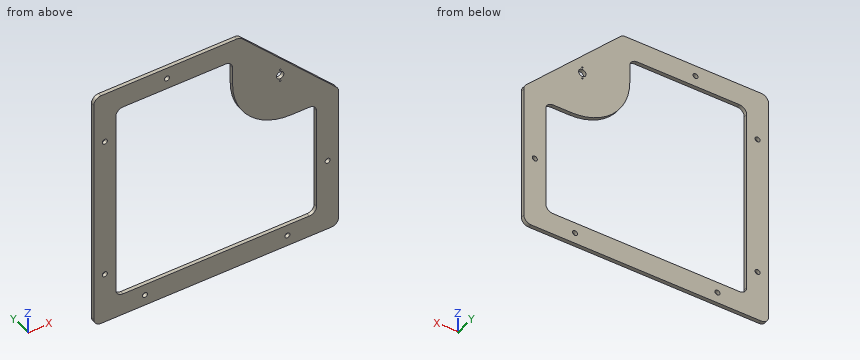
```python
from build123d import *

# Parameters (mm, degrees)
SKETCH1_W                = 425.45
SKETCH1_H                = 425.45
BOSS_EXTRUDE1_DEPTH      = 3.175
CUT_EXTRUDE1_DEPTH       = 301.90558943
SKETCH3_R                = 6.477
SKETCH3_R_2              = 1.27
CUT_EXTRUDE2_DEPTH       = 301.90558943
F_0_332_DIAMETER_HOLE1_D = 8.8392
CUT_EXTRUDE3_DEPTH       = 301.90558943
FILLET1_R                = 12.7
FILLET2_R                = 101.6


with BuildPart() as part:
    # Sketch1 → Boss-Extrude1 (new, symmetric)
    with BuildSketch(Plane(origin=(0, 0, 0), x_dir=(1, 0, 0), z_dir=(0, 1, 0))):
        Rectangle(SKETCH1_W, SKETCH1_H)
    extrude(amount=BOSS_EXTRUDE1_DEPTH, both=True)

    # Sketch2 → Cut-Extrude1 (cut, through all)
    with BuildSketch(Plane(origin=(0, 3.175, 0), x_dir=(1, 0, 0), z_dir=(0, 1, 0))):
        Polygon((212.725, -212.725), (212.725, -41.275), (41.275, -212.725), align=None)
    extrude(amount=-CUT_EXTRUDE1_DEPTH, mode=Mode.SUBTRACT)

    # Sketch3 → Cut-Extrude2 (cut, through all)
    with BuildSketch(Plane(origin=(0, 3.175, 0), x_dir=(1, 0, 0), z_dir=(0, 1, 0))):
        with Locations(Location((111.125, -111.125, 0), (0, 0, 270))):
            Circle(SKETCH3_R)
        with Locations(Location((111.125, -100.7999, 0), (0, 0, 270))):
            Circle(SKETCH3_R_2)
        with Locations(Location((111.125, -121.4501, 0), (0, 0, 270))):
            Circle(SKETCH3_R_2)
    extrude(amount=-CUT_EXTRUDE2_DEPTH, mode=Mode.SUBTRACT)

    # 0.332_ Diameter Hole1 (through all)
    with Locations(Plane(origin=(0, 3.175, 0), x_dir=(1, 0, 0), z_dir=(0, 1, 0))):
        with Locations((-85.725, -193.675), (-193.675, -123.825), (-193.675, 123.825), (-123.825, 193.675), (123.825, 193.675), (193.675, 85.725)):
            Hole(F_0_332_DIAMETER_HOLE1_D / 2)

    # Sketch6 → Cut-Extrude3 (cut, through all)
    with BuildSketch(Plane(origin=(0, 3.175, 0), x_dir=(1, 0, 0), z_dir=(0, 1, 0))):
        Polygon((174.625, 174.625), (174.625, -28.575), (28.575, -28.575), (28.575, -174.625), (-174.625, -174.625), (-174.625, 174.625), align=None)
    extrude(amount=-CUT_EXTRUDE3_DEPTH, mode=Mode.SUBTRACT)

    # Fillet1
    fillet1_edges = [part.edges().sort_by_distance(p)[0] for p in [
        (41.275, 0, 212.725),
        (212.725, 0, 41.275),
        (-212.725, 0, 212.725),
        (-212.725, 0, -212.725),
        (-174.625, 0, -174.625),
        (212.725, 0, -212.725),
        (174.625, 0, -174.625),
        (174.625, 0, 28.575),
        (28.575, 0, 174.625),
        (-174.625, 0, 174.625),
    ]]
    fillet(fillet1_edges, radius=FILLET1_R)

    # Fillet2
    fillet2_edges = [part.edges().sort_by_distance(p)[0] for p in [
        (28.575, 0, 28.575),
    ]]
    fillet(fillet2_edges, radius=FILLET2_R)


solid = part.part
```
Model file for the job. Use its own axes, mm. Give positions to 0.01 mm unless a question says otherwise; leave off trailing zeros. Order: outer loops, then holes, each group sorted by start corner. A loop starts at its lowest first (then second) coordinate and runs counter-clockwise, first axis right, second up.
1) Saw through at B-B, the plane z = 8. Write the cut outline in (x, y) (3 decimals).
2) Pin check, flat tips, straight feed: pin 1 (3 mm diameter, centred on y = -1.5, z = 41.5, fed in from +X); pin 2 (2 mm diameter, centred on x = 41, y = 0, fed in from +Z); pin 3 (1.5 mm diameter, centred on x = 111.12, z = 100.8, fed in from +Y); pin 4 (1 mm diameter, centred on y = -1, z = 100.5, fed in from +X). Stop position of each tip, or through.
3) Saw through at C-C, the plane y = 0.75. Count the separate pieces of the cut face and the enclosed holes in it, then the cut area to 3 significant figures.
4) Saw through at A-A, the plane x = -35.5. Write the cut outline in (y, z) (3 decimals).
5) Wall check: probe 1 along Z at (x, y) = (-85, 1) (3 decimals); probe 2 along X at (y, z) = (-2, -16) (3 decimals). Give the ranges that are in metal, low to high.
Computed:
1. outline: (-212.725, -3.175) - (-174.625, -3.175) - (-174.625, 3.175) - (-212.725, 3.175) - close; (174.625, -3.175) - (212.725, -3.175) - (212.725, 3.175) - (174.625, 3.175) - close
2. pin 1: stops at x = 212.08
2. pin 2: stops at z = 212.08
2. pin 3: passes through
2. pin 4: stops at x = 154
3. separate pieces: 1
3. enclosed holes: 10
3. area: 63,000 mm2
4. outline: (-3.175, -212.725) - (3.175, -212.725) - (3.175, -174.625) - (-3.175, -174.625) - close; (-3.175, 174.625) - (3.175, 174.625) - (3.175, 212.725) - (-3.175, 212.725) - close
5. probe 1: z = -212.725 to -174.625, 174.625 to 189.315, 198.035 to 212.725
5. probe 2: x = -212.725 to -174.625, 174.625 to 212.725
